```python
from build123d import *

# Parameters (mm, degrees)
SCHIZZO1_W                   = 10
SCHIZZO1_H                   = 40
ESTRUSIONE_ESTRUSIONE1_DEPTH = 9
SCHIZZO2_W                   = 10
SCHIZZO2_H                   = 20
TAGLIO_ESTRUSIONE1_DEPTH     = 8
FORO_PER_VITE_M2_1_D         = 2.4
FORO_PER_VITE_M2_1_DEPTH     = 6
FORO_PER_VITE_M2_1_TIP       = 0.721032743
FORO_PER_VITE_M2_2_D         = 7.2


with BuildPart() as part:
    # Schizzo1 → Estrusione-Estrusione1 (new body)
    with BuildSketch(Plane(origin=(0, 0, 0), x_dir=(1, 0, 0), z_dir=(0, 1, 0))):
        Rectangle(SCHIZZO1_W, SCHIZZO1_H)
    extrude(amount=ESTRUSIONE_ESTRUSIONE1_DEPTH)

    # Schizzo2 → Taglio-Estrusione1 (cut)
    with BuildSketch(Plane(origin=(0, 9, 0), x_dir=(1, 0, 0), z_dir=(0, 1, 0))):
        Rectangle(SCHIZZO2_W, SCHIZZO2_H)
    extrude(amount=-TAGLIO_ESTRUSIONE1_DEPTH, mode=Mode.SUBTRACT)

    # Foro per Vite M2-1
    with Locations(Plane(origin=(0, 9, 0), x_dir=(1, 0, 0), z_dir=(0, 1, 0))):
        with Locations((0, -15), (0, 15)):
            Hole(FORO_PER_VITE_M2_1_D / 2, depth=FORO_PER_VITE_M2_1_DEPTH)
            with Locations((0, 0, -(FORO_PER_VITE_M2_1_DEPTH + FORO_PER_VITE_M2_1_TIP / 2))):  # 118° drill point
                Cone(0, FORO_PER_VITE_M2_1_D / 2, FORO_PER_VITE_M2_1_TIP, mode=Mode.SUBTRACT)

    # Foro per Vite M2-2 (through all)
    with Locations(Plane(origin=(0, 1, 0), x_dir=(1, 0, 0), z_dir=(0, 1, 0))):
        with Locations((0, 0)):
            Hole(FORO_PER_VITE_M2_2_D / 2)


solid = part.part
```
Source: CAD feature listing. Evaluate the final solid. Frame: model axes, mm. A direction names the side the tool comes from. Coordinates: 2 decimals unless noted, no trailing zeros. Loops run counter-clockwise (first coordinate to the right, second up) from the corner with the lowest first, then second, coordinate; pieces in that order, holes last. Notation, with made-up numbers: M -13.75,14 L 26.25,14 A23 ccw 26.25,25 Z; hole C 40.5,77 d10. An arc over 180 degrees is marked long. Use a Markdown table: item, result. Add a question column.
Q1. First-contact query: pin 1 (3 mm diameter, centred on x = -2, z = -2.5, fed in from +Y). Flat tip, straight axial feed; report the tip coordinate or a pass-through.
Q2. Section query C-C, the plane x = -1.75. Return loops of the section in (y, z).
Q3. Section query B-B, the plane y = 1.75. Return loops of the section in (x, z), and give its area (3 significant figures).
Q4. Material intervals for L1, parallel to Z at x = -2.25, y = 3.75; L2, parallel to Z at x = -0.25, y = 7.75; L3, parallel to X at y = 6.1, z = -15, sorted ascending.
Q5. Section query D-D, the plane z = -9. Return loops of the section in (x, y), and give its area (3 significant figures).
Q6. Access query for faces 5 (the cylindrical face through (-0.554, 5.958, 16.065)), 6 (the flat face through (5, 0.4, 0.3)), 7 (the flat face through (0, 5, 10)). Directions: +Z, -Z, +X, -X, +Y, -Y. A direction counts if a zero-diameter tool reaches every point of the face in a straight line with its end or side. Return the directions, or none.
Q7. Section query A-A, the plane z = 0. Return loops of the section in (x, y).
Q8. Draft query along Z for faces 1 (the flat face through (0, 4, 20)), 2 (the flat face through (-1, 9, -14)), 3 (the flat face through (0, 5, -10)), 4 (the flat face through (0, 4, -20)). Return one class per face: pulls with the +Z half, pulls with the -Z half, needs draft (parallel to the pull), parting line crosses it, or undercut.
Result:
| question | item | result |
|---|---|---|
| 1 | pin 1 | stops at y = 1 |
| 2 | outline | M 0,-20 L 9,-20 L 9,-10 L 1,-10 L 1,-3.15 L 0,-3.15 Z; M 0,3.15 L 1,3.15 L 1,10 L 9,10 L 9,20 L 0,20 Z |
| 3 | outline | M -5,-20 L 5,-20 L 5,-10 L -5,-10 Z; M -5,10 L 5,10 L 5,20 L -5,20 Z |
| 3 | area | 200 mm2 |
| 4 | L1 | z = -20 to -10, 10 to 20 |
| 4 | L2 | z = -20 to -16.17, -13.83 to -10, 10 to 13.83, 16.17 to 20 |
| 4 | L3 | x = -5 to -1.2, 1.2 to 5 |
| 5 | outline | M -5,0 L 5,0 L 5,1 L -5,1 Z |
| 5 | area | 10.0 mm2 |
| 6 | face 5 | +Y |
| 6 | face 6 | +Z, -Z, +X, +Y, -Y |
| 6 | face 7 | +X, -X, +Y |
| 7 | outline | M -5,0 L -3.6,0 L -3.6,1 L -5,1 Z; M 3.6,0 L 5,0 L 5,1 L 3.6,1 Z |
| 8 | face 1 | pulls with the +Z half |
| 8 | face 2 | needs draft |
| 8 | face 3 | undercut |
| 8 | face 4 | pulls with the -Z half |
